```python
from build123d import *

# Parameters (mm, degrees)
SKETCH1_W           = 200
SKETCH1_H           = 100
BOSS_EXTRUDE1_DEPTH = 10
SKETCH2_R           = 7.5
SKETCH2_R_2         = 13.5
SKETCH2_R_3         = 10
SKETCH2_W           = 50
SKETCH2_H           = 35
CUT_EXTRUDE1_DEPTH  = 114.578166916


with BuildPart() as part:
    # Sketch1 → Boss-Extrude1 (new, symmetric)
    with BuildSketch(Plane(origin=(0, 0, 0), x_dir=(1, 0, 0), z_dir=(0, 1, 0))):
        Rectangle(SKETCH1_W, SKETCH1_H)
    extrude(amount=BOSS_EXTRUDE1_DEPTH, both=True)

    # Sketch2 → Cut-Extrude1 (cut, through all)
    with BuildSketch(Plane(origin=(0, 10, 0), x_dir=(1, 0, 0), z_dir=(0, 1, 0))):
        with Locations(Location((-80, 30, 0), (0, 0, 270))):
            Circle(SKETCH2_R)
        with Locations(Location((-55, 0, 0), (0, 0, 270))):
            Circle(SKETCH2_R_2)
        with Locations(Location((75, 20, 0), (0, 0, 270))):
            Circle(SKETCH2_R_3)
        with Locations(Location((45, -35, 0), (0, 0, 270))):
            Circle(SKETCH2_R_3)
        Rectangle(SKETCH2_W, SKETCH2_H)
    extrude(amount=-CUT_EXTRUDE1_DEPTH, mode=Mode.SUBTRACT)


solid = part.part
```
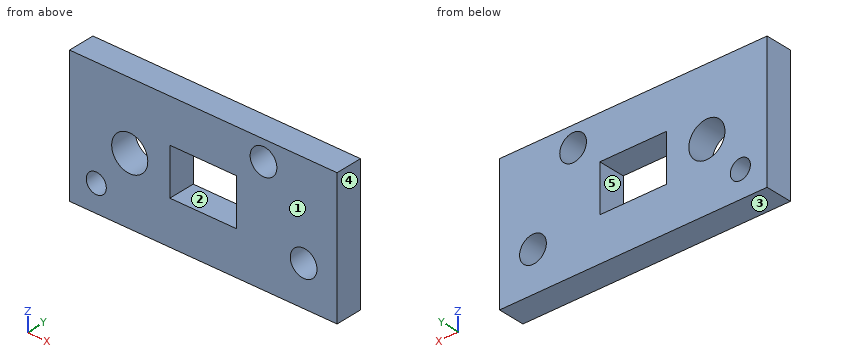
Geometry check sheet. Reference: the model listing, model coordinates, mm. Face numbers are marked on the shaded views. A direction names the side the tool comes from. Give positions to 0.01 mm unless a question says otherwise; leave off trailing zeros. Loops run counter-clockwise (first coordinate to the right, second up) from the corner with the lowest first, then second, coordinate; pieces in that order, holes last. Notation, with made-up numbers: M 34.25,15 L 80.25,15 A14 cw 80.25,20 Z; hole C -16.5,62 d5. An arc over 180 degrees is marked long. Answer as CSV lines item,"result".
Item 1: Release check for a two-part mould opening along X. For the marked faces 3, 4 and 5 record: pulls with the +X half, pulls with the -X half, needs draft (parallel to the pull), parting line crosses it, or undercut.
Values:
face 3,"needs draft"
face 4,"pulls with the +X half"
face 5,"undercut"
Item 2: Cross-section at B-B on z = 35. Record the cut outline in (x, y), and give its area (3 significant figures).
Values:
outline,"M -100,-10 L 35,-10 L 35,10 L -100,10 Z; M 55,-10 L 100,-10 L 100,10 L 55,10 Z"
area,"3,600 mm²"
Item 3: Cross-section at C-C on y = -5. Record the cut outline in (x, z), and give its area (3 significant figures).
Values:
outline,"M -100,-50 L 100,-50 L 100,50 L -100,50 Z; hole C -80,-30 d15; hole C -55,0 d27; hole M -25,-17.5 L 25,-17.5 L 25,17.5 L -25,17.5 Z; hole C 45,35 d20; hole C 75,-20 d20"
area,"16,900 mm²"
Item 4: Cross-section at A-A on x = 75. Record the cut outline in (y, z).
Values:
outline,"M -10,-50 L 10,-50 L 10,-30 L -10,-30 Z; M -10,-10 L 10,-10 L 10,50 L -10,50 Z"
Item 5: Material ranges on line 1 (X direction, y = -5.5, z = -20.5); line 2 (X direction, y = 8, z = 42); line 3 (Z direction, x = -52.5, y = -7.5), recorded low to high.
Values:
line 1,"x = -100 to 65.01, 84.99 to 100"
line 2,"x = -100 to 37.86, 52.14 to 100"
line 3,"z = -50 to -13.27, 13.27 to 50"
Item 6: Access from +Z, -Z, +X, -X, +Y, -Y to the whole of each face (thin tool, end or side, straight path). Record for the marked faces 1 and 2.
Values:
face 1,"+Z, -Z, +X, -X, -Y"
face 2,"+Y, -Y"
Item 7: Cross-section at D-D on z = 0. Record the cut outline in (x, y), and give its area (3 significant figures).
Values:
outline,"M -100,-10 L -68.5,-10 L -68.5,10 L -100,10 Z; M -41.5,-10 L -25,-10 L -25,10 L -41.5,10 Z; M 25,-10 L 100,-10 L 100,10 L 25,10 Z"
area,"2,460 mm²"
